Could you check a few things on this model? Use its own coordinates, in mm. A direction names the side the tool comes from. Give positions to 0.01 mm unless a question says otherwise; leave off trailing zeros. Loops run counter-clockwise (first coordinate to the right, second up) from the corner with the lowest first, then second, coordinate; pieces in that order, holes last. Notation, with made-up numbers: (63, -35) -> (88, -35) arc R22 ccw to (88, -13) -> close; hole circle Ø1 at (59, 60). An arc over 180 degrees is marked (long way). Put each result on its own line as item: value.
```python
from build123d import *

# Parameters (mm, degrees)
SKETCH1_W                                           = 30
SKETCH1_H                                           = 30
MOUNT_BLOCK_DEPTH                                   = 6.35
LINEAR_STAGE_CBORE_FOR_M3_SBHCS1_D                  = 3.4
LINEAR_STAGE_CBORE_FOR_M3_SBHCS1_CBORE_D            = 6.7
LINEAR_STAGE_CBORE_FOR_M3_SBHCS1_CBORE_DEPTH        = 1.65
OPTICAL_POST_CBORE_FOR_8_SOCKET_HEAD_CA_D           = 4.4958
OPTICAL_POST_CBORE_FOR_8_SOCKET_HEAD_CA_CBORE_D     = 7.9375
OPTICAL_POST_CBORE_FOR_8_SOCKET_HEAD_CA_CBORE_DEPTH = 4.1656


with BuildPart() as part:
    # Sketch1 → Mount Block (new body)
    with BuildSketch(Plane(origin=(0, 0, 0), x_dir=(1, 0, 0), z_dir=(0, 1, 0))):
        Rectangle(SKETCH1_W, SKETCH1_H)
    extrude(amount=MOUNT_BLOCK_DEPTH)

    # Linear Stage CBORE for M3 SBHCS1 (through all)
    with Locations(Plane(origin=(0, 6.35, 0), x_dir=(1, 0, 0), z_dir=(0, 1, 0))):
        with Locations((-10, 10), (10, 10), (10, -10.066), (-10, -10.066)):
            CounterBoreHole(LINEAR_STAGE_CBORE_FOR_M3_SBHCS1_D / 2, LINEAR_STAGE_CBORE_FOR_M3_SBHCS1_CBORE_D / 2, LINEAR_STAGE_CBORE_FOR_M3_SBHCS1_CBORE_DEPTH)

    # Optical Post CBORE for #8 Socket Head Cap Screw (through all)
    with Locations(Plane(origin=(0, 0, 0), x_dir=(-1, 0, 0), z_dir=(0, -1, 0))):
        with Locations((0, 0)):
            CounterBoreHole(OPTICAL_POST_CBORE_FOR_8_SOCKET_HEAD_CA_D / 2, OPTICAL_POST_CBORE_FOR_8_SOCKET_HEAD_CA_CBORE_D / 2, OPTICAL_POST_CBORE_FOR_8_SOCKET_HEAD_CA_CBORE_DEPTH)


solid = part.part
```
1. If we section it at A-A (x = 10): List the corners of the cut face in (y, z) for me, then the cut area to 3 significant figures.
Recorded:
outline: (0, -15) -> (6.35, -15) -> (6.35, -13.35) -> (4.7, -13.35) -> (4.7, -11.7) -> (0, -11.7) -> close; (0, -8.3) -> (4.7, -8.3) -> (4.7, -6.65) -> (6.35, -6.65) -> (6.35, 6.72) -> (4.7, 6.72) -> (4.7, 8.37) -> (0, 8.37) -> close; (0, 11.77) -> (4.7, 11.77) -> (4.7, 13.42) -> (6.35, 13.42) -> (6.35, 15) -> (0, 15) -> close
area: 136 mm^2
2. If we section it at D-D (z = -10): List the corners of the cut face in (x, y) for me, then the cut area to 3 significant figures.
Recorded:
outline: (-15, 0) -> (-11.7, 0) -> (-11.7, 4.7) -> (-13.35, 4.7) -> (-13.35, 6.35) -> (-15, 6.35) -> close; (-8.3, 0) -> (8.3, 0) -> (8.3, 4.7) -> (6.65, 4.7) -> (6.65, 6.35) -> (-6.65, 6.35) -> (-6.65, 4.7) -> (-8.3, 4.7) -> close; (11.7, 0) -> (15, 0) -> (15, 6.35) -> (13.35, 6.35) -> (13.35, 4.7) -> (11.7, 4.7) -> close
area: 136 mm^2
3. Thinking about a two-plate mould opening in Z: for faces 1 (the face through (0.86, 2.054, 3.874)), 2 (the face through (-10.436, 5.537, 6.745)), 3 (the face through (15, 3, 0)), 4 (the face through (0, 3, 15)), which applies, pulls with the +Z half, pulls with the -Z half, needs draft (parallel to the pull), parting line crosses it, or undercut?
Recorded:
face 1: undercut
face 2: undercut
face 3: needs draft
face 4: pulls with the +Z half
4. If we section it at C-C (x = 0): List the corners of the cut face in (y, z) for me.
Recorded:
outline: (0, -15) -> (6.35, -15) -> (6.35, -2.25) -> (4.17, -2.25) -> (4.17, -3.97) -> (0, -3.97) -> close; (0, 3.97) -> (4.17, 3.97) -> (4.17, 2.25) -> (6.35, 2.25) -> (6.35, 15) -> (0, 15) -> close
5. I need wall thicknesses on line 1 (Z direction, x = -10, y = 1.2); line 2 (Z direction, x = 0, y = 5.9); line 3 (Z direction, x = 9, y = 2.5). Which ranges of each line are inside material? Lowest first, please.
Recorded:
line 1: z = -15 to -11.7, -8.3 to 8.37, 11.77 to 15
line 2: z = -15 to -2.25, 2.25 to 15
line 3: z = -15 to -11.37, -8.63 to 8.69, 11.44 to 15
6. If we section it at B-B (z = 0): List the corners of the cut face in (x, y) for me.
Recorded:
outline: (-15, 0) -> (-3.97, 0) -> (-3.97, 4.17) -> (-2.25, 4.17) -> (-2.25, 6.35) -> (-15, 6.35) -> close; (2.25, 4.17) -> (3.97, 4.17) -> (3.97, 0) -> (15, 0) -> (15, 6.35) -> (2.25, 6.35) -> close
7. For faces 5 (the face through (9.09, 2.32, 8.63)), 6 (the face through (8, 4.7, 9)), which set-ups out of +Z, -Z, +X, -X, +Y, -Y let a thin tool reach every point of the face, with its end or its side?
Recorded:
face 5: +Y, -Y
face 6: +Y
8. I'm going to push flat-ended pins straight in: pin 1 (2 mm diameter, centred on x = 8.5, z = 10.5, fed in from +Y); pin 2 (2.5 mm diameter, centred on x = -1, z = 1.5, fed in from -Y). Where does each tip first touch, or does it pass through?
Recorded:
pin 1: stops at y = 4.7
pin 2: stops at y = 4.17
